Geometry: final body of the model. Coordinates: model frame, mm. A direction names the side the tool comes from. Coordinates: 2 decimals unless noted, no trailing zeros. Write each loop counter-clockwise with the first axis right and the second up, starting at its lowest first coordinate (ties: lowest second). Pieces come first, ordered by that corner, then holes. Notation, with made-up numbers: (23.25, 32) -> (77.25, 32) arc R24 cw to (77.25, 44) -> close; hole circle Ø5 at (47, 39.25). An arc over 180 degrees is marked (long way). One line per item, written item: value.
```python
from build123d import *

# Parameters (mm, degrees)
BOSS_EXTRUDE3_DEPTH       = 70
BOSS_EXTRUDE4_DEPTH       = 90
M8_TAPPED_HOLE2_D         = 6.8
MIRROR5_COPY_1_D          = 6.8
M8X1_0_TAPPED_HOLE1_D     = 7
M8X1_0_TAPPED_HOLE1_DEPTH = 11
M8X1_0_TAPPED_HOLE1_TIP   = 2.103012167
M8X1_0_TAPPED_HOLE2_D     = 7
M8X1_0_TAPPED_HOLE2_DEPTH = 11
M8X1_0_TAPPED_HOLE2_TIP   = 2.103012167


with BuildPart() as part:
    # Sketch2 → Boss-Extrude3 (new, symmetric)
    with BuildSketch(Plane.XY):
        with BuildLine():
            ThreePointArc((-61, 30), (-62.647726429, 13.739490403), (-71.499030185, 0))
            Line((-71.499030185, 0), (244, 0))
            Line((244, 0), (244, 30))
            Line((244, 30), (-61, 30))
        make_face()
        with BuildLine():
            Line((244, 30), (244, 0))
            Line((244, 0), (559.499030185, 0))
            ThreePointArc((559.499030185, 0), (550.647726429, 13.739490403), (549, 30))
            Line((549, 30), (244, 30))
        make_face()
    extrude(amount=BOSS_EXTRUDE3_DEPTH, both=True)

    # Sketch2<3> → Boss-Extrude4 (add, symmetric)
    with BuildSketch(Plane.XY):
        with BuildLine():
            Line((585.195897576, 60.268095002), (583.196848208, 53.296581361))
            ThreePointArc((583.196848208, 53.296581361), (556.31388494, 31.210623184), (571.688547964, 0))
            Line((571.688547964, 0), (559.499030185, 0))
            ThreePointArc((559.499030185, 0), (551.487488703, 39.028239626), (585.195897576, 60.268095002))
        make_face()
        with BuildLine():
            Line((-83.688547964, 0), (-71.499030185, 0))
            ThreePointArc((-71.499030185, 0), (-63.487488703, 39.028239626), (-97.195897576, 60.268095002))
            Line((-97.195897576, 60.268095002), (-95.196848208, 53.296581361))
            ThreePointArc((-95.196848208, 53.296581361), (-68.31388494, 31.210623184), (-83.688547964, 0))
        make_face()
    extrude(amount=BOSS_EXTRUDE4_DEPTH, both=True)

    # M8 Tapped Hole2 (through all)
    with Locations(Plane(origin=(560.080057986, 40.36388188, 50), x_dir=(0.537967071811, 0.842965853191, 0), z_dir=(0.842965853191, -0.537967071811, 0))):
        with Locations((1e-09, 0)):
            m8_tapped_hole2 = Hole(M8_TAPPED_HOLE2_D / 2)

    # Mirror4: M8 Tapped Hole2 across plane
    add(m8_tapped_hole2.mirror(Plane.XY), mode=Mode.SUBTRACT)

    # Mirror5: M8 Tapped Hole2 across plane
    add(m8_tapped_hole2.mirror(Plane.ZY.offset(-244)), mode=Mode.SUBTRACT)

    # Mirror5 copy 1 (through all)
    with Locations(Plane(origin=(-72.080057986, 40.36388188, -50), x_dir=(-0.5379670718110001, 0.8429658531909999, 0), z_dir=(-0.8429658531909999, -0.5379670718110001, 0))):
        with Locations((1e-09, 0)):
            Hole(MIRROR5_COPY_1_D / 2)

    # M8x1.0 Tapped Hole1
    with Locations(Plane(origin=(0, 30, 0), x_dir=(1, 0, 0), z_dir=(0, 1, 0))):
        with Locations((425, 25), (425, -25)):
            Hole(M8X1_0_TAPPED_HOLE1_D / 2, depth=M8X1_0_TAPPED_HOLE1_DEPTH)
            with Locations((0, 0, -(M8X1_0_TAPPED_HOLE1_DEPTH + M8X1_0_TAPPED_HOLE1_TIP / 2))):  # 118° drill point
                Cone(0, M8X1_0_TAPPED_HOLE1_D / 2, M8X1_0_TAPPED_HOLE1_TIP, mode=Mode.SUBTRACT)

    # M8x1.0 Tapped Hole2
    with Locations(Plane(origin=(0, 30, 0), x_dir=(1, 0, 0), z_dir=(0, 1, 0))):
        with Locations((-25, 25), (-25, -25)):
            Hole(M8X1_0_TAPPED_HOLE2_D / 2, depth=M8X1_0_TAPPED_HOLE2_DEPTH)
            with Locations((0, 0, -(M8X1_0_TAPPED_HOLE2_DEPTH + M8X1_0_TAPPED_HOLE2_TIP / 2))):  # 118° drill point
                Cone(0, M8X1_0_TAPPED_HOLE2_D / 2, M8X1_0_TAPPED_HOLE2_TIP, mode=Mode.SUBTRACT)


solid = part.part
```
(1) First-contact query: pin 1 (9 mm diameter, centred on x = 329, y = 12, fed in from -Z); pin 2 (12 mm diameter, centred on x = 293, y = 28, fed in from +Z); pin 3 (5 mm diameter, centred on y = 14.5, z = -70.5, fed in from +X). Flat tips, straight axial feed; report the tip coordinate or a pass-through.
Responses:
pin 1: stops at z = -70
pin 2: stops at z = 70
pin 3: stops at x = 559.04
(2) Section B-B (x = 233.5). Return the cut outline in (y, z), then the cut area to 3 significant figures.
Responses:
outline: (0, -70) -> (30, -70) -> (30, 70) -> (0, 70) -> close
area: 4,200 mm2
(3) Line query: line 1 (X direction, y = 25, z = -25); line 2 (Z direction, x = -25, y = 25.75); line 3 (X direction, y = 27.5, z = -25). Output: solid intervals per line, ascending. Write a range as [from, to].
Responses:
line 1: x = [-67.68, -28.5], [-21.5, 421.5], [428.5, 555.68]
line 2: z = [-70, -28.5], [-21.5, 21.5], [28.5, 70]
line 3: x = [-67.77, -28.5], [-21.5, 421.5], [428.5, 555.77]
(4) Section A-A (z = -7.5). Return the cut outline in (x, y), then the cut area to 3 significant figures.
Responses:
outline: (-97.2, 60.27) -> (-95.2, 53.3) arc R28 cw to (-83.69, 0) -> (571.69, 0) arc R28 cw to (583.2, 53.3) -> (585.2, 60.27) arc R35 ccw to (549, 30) -> (-61, 30) arc R35 ccw to start
area: 19,600 mm2
(5) Pull-direction query (X, two-part tool) for faces 1 (the flat face through (240, 15, 70)), 2 (the cylindrical face through (-68.43, 31.72, 1.26)), 3 (the flat face through (-68, 33, -90)); classes: released by +X, released by -X, zero draft, split by the parting line, or undercut.
Responses:
face 1: undercut
face 2: released by -X
face 3: zero draft
(6) Reachability of faces 4 (the flat face through (248, 30, 1)), 5 (the flat face through (556, 33, -90)) from +Z, -Z, +X, -X, +Y, -Y: full face, straight path, thin tool, end or side. Return the list, or none.
Responses:
face 4: +Z, -Z, +Y
face 5: -Z, +X, -X, +Y, -Y
